Autodesk Inventor part; units mm, degrees
ref_plane "YZ Plane" through (0, 0, 0) normal (1, 0, 0) x (0, 1, 0)
ref_plane "XZ Plane" through (0, 0, 0) normal (0, 1, 0) x (-1, 0, 0)
ref_plane "XY Plane" through (0, 0, 0) normal (0, 0, 1) x (1, 0, 0)
sketch "Skizze1" plane through (0, 0, 0) normal (0, 0, 1) x (1, 0, 0)
  line L0 (-15.4, 0) -> (15.4, 0)
  line L1 (0, -15.4) -> (0, 15.4)
  circle A0 centre (0, 0) radius 11
  circle A1 centre (0, 0) radius 4
  dimension "d0" = 22
  dimension "d1" = 8
extrude "Extrusion1" add sketch "Skizze1" along normal mid plane 7 contours A1 L1 A0 L0 | L0 A0 L1 A1 | A1 L0 A0 L1 | L1 A0 L0 A1
sketch "Skizze2" plane through (0, 0, 3.5) normal (0, 0, 1) x (1, 0, 0)
  circle A0 centre (0, 0) radius 4
  circle A1 centre (0, 0) radius 11
  circle A2 centre (0, 0) radius 5
  circle A3 centre (0, 0) radius 10
  dimension "d4" = 10
  dimension "d5" = 20
extrude "Extrusion2" cut sketch "Skizze2" against normal blind 0.2 contours A3
mirror "Spiegeln1" about plane through (0, 0, 0) normal (0, 0, 1) of "Extrusion2"
chamfer "Fase1" distance 0.05 angle 45 1 edges at (-10, 0, 3.5)
chamfer "Fase2" distance 0.05 angle 45 1 edges at (-5, 0, 3.5)
chamfer "Fase3" distance 0.05 angle 45 1 edges at (-4, 0, 3.5)
chamfer "Fase4" distance 0.05 angle 45 1 edges at (-11, 0, 3.5)
chamfer "Fase5" distance 0.05 angle 45 1 edges at (-11, 0, -3.5)
chamfer "Fase6" distance 0.05 angle 45 1 edges at (-10, 0, -3.5)
chamfer "Fase7" distance 0.05 angle 45 1 edges at (-5, 0, -3.5)
chamfer "Fase8" distance 0.05 angle 45 1 edges at (-4, 0, -3.5)
properties part number "Kugellager_8x22x7_608ZZ" material "Stahl, Kohlenstoff"
Model file for the job. Use its own axes, mm. A direction names the side the tool comes from. Give positions to 0.01 mm unless a question says otherwise; leave off trailing zeros. Write each loop counter-clockwise with the first axis right and the second up, starting at its lowest first coordinate (ties: lowest second). Pieces come first, ordered by that corner, then holes. Notation, with made-up numbers: (76.5, 7) -> (84.5, 7) arc R13 cw to (84.5, 16) -> close; hole circle Ø5 at (67.5, 32.25). An arc over 180 degrees is marked (long way). Write item = value, one per line.
(1) Mould opens along Y. For faces 3 (the face through (-2.38, -10.74, 0.05)), 4 (the face through (5, -9, 3.5)), 5 (the face through (2, 5, 3.3)) say: released by +Y, released by -Y, zero draft, split by the parting line, or undercut.
Determined:
face_3 = split by the parting line
face_4 = zero draft
face_5 = undercut
(2) Tool access for faces 1 (the face through (-2, 5, -3.3)), 2 (the face through (-2, -4, 3.5)): list every direction of +Z, -Z, +X, -X, +Y, -Y with a clear straight run to the whole face (end or side of a thin tool).
Determined:
face_1 = -Z
face_2 = +Z, +X, -X, +Y, -Y
(3) Probe line 1 along X through (y, z) = (0, -1.75); line 2 along Y through (x, z) = (0, -3.35). List the from-to ranges inside material, lowest first.
Determined:
line_1 = -11 to -4, 4 to 11
line_2 = -11 to -10, -5 to -4, 4 to 5, 10 to 11
(4) Flat gauge pins, fed straight in: P1, Ø1.5, axis at y = 3.5, z = -1.5, coming from the +X side; P2, Ø13, axis at x = 0, y = 0, coming from the -Z side; P3, Ø2, axis at y = -2.5, z = 1, coming from the -X side; P4, Ø3, axis at x = 2, z = -2, coming from the +Y side. Where does each tip first touch, or does it go through?
Determined:
P1 = 10.65
P2 = -3.5
P3 = -10.9
P4 = 10.99
(5) Slice it at A-A, the plane z = -0.75. Give the cut face in (x, y), then the cut area to 3 significant figures.
Determined:
outline = circle Ø22 at (0, 0); hole circle Ø8 at (0, 0)
area = 330 mm2
